```python
from build123d import *

# Parameters (mm, degrees)
F1_DEPTH      = 9
F0_W          = 10
F0_H          = 64
F2_DEPTH      = 56
F0_W_2        = 22
F0_H_2        = 25
F3_DEPTH      = 35
F4_DEPTH      = 12
F4_DEPTH_BACK = 10
F5_W          = 14
F5_H          = 25
F6_DEPTH      = 16


with BuildPart() as f1:
    # F0 (on Top) → F1 (new body)
    with BuildSketch(Plane.XY):
        with BuildLine():
            Line((-143, 22), (-143, -42))
            Line((-143, -42), (-86, -42))
            ThreePointArc((-86, -42), (-77.6864285452, -21.1714486497), (-57.0043106652, -12.5))
            Line((-57.0043106652, -12.5), (0, -12.5))
            ThreePointArc((0, -12.5), (-12.4769155686, 0.7593272639), (1.5158499456, 12.407747537))
            Line((1.5158499456, 12.407747537), (-77, 22))
            Line((-77, 22), (-77, -3))
            Line((-77, -3), (-99, -3))
            Line((-99, -3), (-99, 22))
            Line((-99, 22), (-143, 22))
        make_face()
    extrude(amount=F1_DEPTH)

    # F0 (on Top) → F2 (join)
    with BuildSketch(Plane.XY):
        with Locations((-148, -10)):
            Rectangle(F0_W, F0_H)
    extrude(amount=F2_DEPTH)

    # F0 (on Top) → F3 (join)
    with BuildSketch(Plane.XY):
        with Locations((-88, 9.5)):
            Rectangle(F0_W_2, F0_H_2)
    extrude(amount=F3_DEPTH)

    # F0 (on Top) → F4 (join, two sides)
    with BuildSketch(Plane.XY) as f4_sk:
        with BuildLine():
            ThreePointArc((1.5158499456, 12.407747537), (-12.4769155686, 0.7593272639), (0, -12.5))
            ThreePointArc((0, -12.5), (8.8388347648, -8.8388347648), (12.5, 0))
            ThreePointArc((12.5, 0), (9.3594370643, 8.2855861494), (1.5158499456, 12.407747537))
        make_face()
    extrude(amount=F4_DEPTH)
    extrude(f4_sk.sketch, amount=-F4_DEPTH_BACK)

    # F5 (on face) → F6 (join)
    with BuildSketch(Plane.XY.offset(35)):
        with Locations((-84, 9.5)):
            Rectangle(F5_W, F5_H)
    extrude(amount=-F6_DEPTH)


solid = f1.part
```
Model file for the job. Use its own axes, mm. A direction names the side the tool comes from. Coordinates: 2 decimals unless noted, no trailing zeros. Order: outer loops, then holes, each group sorted by start corner. A loop starts at its lowest first (then second) coordinate and runs counter-clockwise, first axis right, second up. Notation, with made-up numbers: (40.25, 59) - (58.25, 59) arc R20 cw to (58.25, 88) - close; hole circle Ø7 at (-2.5, 1.25). An arc over 180 degrees is marked (long way). Return JSON: item names as keys, results as strings. Group by question number.
1) Saw through at D-D, the plane x = -114. Write the cut outline in (y, z), plus the area to 3 significant figures.
2) Saw through at A-A, the plane z = 20. Write the cut outline in (x, y).
3) Probe line 1 (X direction, y = -5.5, z = 48.5); line 2 (Z direction, x = -51.5, y = -0.5); line 3 (Z direction, x = 0, y = 1.5). List the from-to ranges inside material, lowest first. Write a range as from..to.
4) Saw through at C-C, the plane z = 2. Write the cut outline in (x, y).
5) Flat gauge pins, fed straight in: P1, Ø6.5, axis at x = -87, z = 28.5, coming from the -Y side; P2, Ø6, axis at y = -22.5, z = 15, coming from the +X side; P3, Ø5, axis at x = -94.5, y = -7.5, coming from the -Z side. Where does each tip first touch, or does it go through?
6) Tool access for faces 4 (the flat face through (-88, 10, 35)), 5 (the flat face through (0, 0, -10)), 6 (the flat face through (-29, -12.5, 4)), 7 (the flat face through (-143, -10, 32)), 8 (the flat face through (-153, -10, 28)): list every direction of +Z, -Z, +X, -X, +Y, -Y with a clear straight run to the whole face (end or side of a thin tool).
7) Saw through at B-B, the plane y = 0. Write the cut outline in (x, z).
8) Mould opens along X. For faces 1 (the flat face through (-94, -2, 0)), 2 (the flat face through (-37.192, 17.137, 4.437)), 3 (the flat face through (-99, 9, 22)) say: released by +X, released by -X, zero draft, split by the parting line, or undercut.
Values found:
{
 "1": {"outline": "(-42, 0) - (22, 0) - (22, 9) - (-42, 9) - close", "area": "576 mm²"},
 "2": {"outline": "(-153, -42) - (-143, -42) - (-143, 22) - (-153, 22) - close; (-99, -3) - (-77, -3) - (-77, 22) - (-99, 22) - close"},
 "3": {"line 1": "x = -153..-143", "line 2": "z = 0..9", "line 3": "z = -10..12"},
 "4": {"outline": "(-153, -42) - (-86, -42) arc R29 cw to (-57, -12.5) - (0, -12.5) arc R12.5 ccw to (1.52, 12.41) - (-77, 22) - (-153, 22) - close"},
 "5": {"P1": "stops at y = -3", "P2": "stops at x = -143", "P3": "stops at z = 0"},
 "6": {"face 4": "+Z, +X, +Y, -Y", "face 5": "-Z, +X, -X, +Y, -Y", "face 6": "+Z, -Z, +X, -Y", "face 7": "+Z, +Y, -Y", "face 8": "+Z, -Z, -X, +Y, -Y"},
 "7": {"outline": "(-153, 0) - (-12.5, 0) - (-12.5, -10) - (12.5, -10) - (12.5, 12) - (-12.5, 12) - (-12.5, 9) - (-77, 9) - (-77, 35) - (-99, 35) - (-99, 9) - (-143, 9) - (-143, 56) - (-153, 56) - close"},
 "8": {"face 1": "zero draft", "face 2": "released by +X", "face 3": "undercut"}
}
